from build123d import *

# Parameters (mm, degrees)
F1_DEPTH = 38.1
F2_R     = 19.05
F3_DEPTH = 101.601


with BuildPart() as f1:
    # F0 (on Top) → F1 (new body, symmetric)
    with BuildSketch(Plane.XY):
        Polygon((-50.8, -25.4), (50.8, -25.4), (50.8, 25.4), (25.4, 25.4), (0, 25.4), (-25.4, 25.4), (-50.8, 25.4), align=None)
        Polygon((0, 25.4), (25.4, 25.4), (25.4, 76.2), (-25.4, 76.2), (-25.4, 25.4), align=None)
    extrude(amount=F1_DEPTH, both=True)

    # F2 (on face) → F3 (cut, through all)
    with BuildSketch(Plane.YZ.offset(50.8)):
        Circle(F2_R)
    extrude(amount=-F3_DEPTH, mode=Mode.SUBTRACT)


solid = f1.part
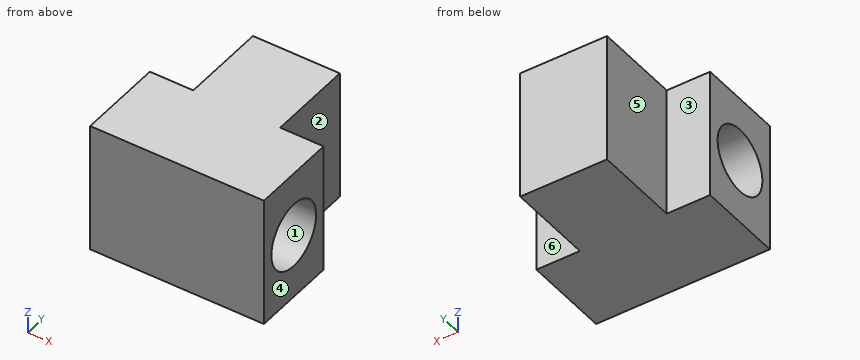
The model under review builds one solid part; all positions refer to its coordinate system, in mm. Face numbers are marked on the shaded views. A direction names the side the tool comes from. Round coordinates to 2 decimals unless told otherwise and drop trailing zeros. Order: outer loops, then holes, each group sorted by start corner. A loop starts at its lowest first (then second) coordinate and runs counter-clockwise, first axis right, second up. Notation, with made-up numbers: (83, -12) - (112, -12) arc R23 cw to (112, 4) - close; hole circle Ø7 at (27.25, 68). An arc over 180 degrees is marked (long way). Use one line per item in the form item = value.
Q1. Add section B-B on y = 0. Give the boundary of the cut face in (x, z), then the cut area to 3 significant figures.
Response values:
outline = (-50.8, -38.1) - (50.8, -38.1) - (50.8, -19.05) - (-50.8, -19.05) - close; (-50.8, 19.05) - (50.8, 19.05) - (50.8, 38.1) - (-50.8, 38.1) - close
area = 3,870 mm^2
Q2. To check wall thickness, follow line 1 (Z direction, x = -23, y = 0); line 2 (X direction, y = 43.5, z = 29); line 3 (Z direction, x = 14.5, y = -9). State the ranges of each line that lie inside material, in increasing order.
Response values:
line_1 = -38.1 to -19.05, 19.05 to 38.1
line_2 = -25.4 to 25.4
line_3 = -38.1 to -16.79, 16.79 to 38.1
Q3. Add section C-C on x = 5.5. Give the boundary of the cut face in (y, z), then the cut area to 3 significant figures.
Response values:
outline = (-25.4, -38.1) - (76.2, -38.1) - (76.2, 38.1) - (-25.4, 38.1) - close; hole circle Ø38.1 at (0, 0)
area = 6,600 mm^2
Q4. Tool access review of the marked faces 4, 5 and 6: name each direction out of +Z, -Z, +X, -X, +Y, -Y from which nothing blocks a thin tool from reaching the whole face with its end or side.
Response values:
face_4 = +Z, -Z, +X, +Y, -Y
face_5 = +Z, -Z, -X, +Y
face_6 = +Z, -Z, +X, +Y
Q5. Clearance check with flat-ended pins moving along their axes: P1, Ø15, axis at y = 49.5, z = -13.5, coming from the +X side; P2, Ø1.5, axis at y = -1, z = 17, coming from the +X side; P3, Ø12.5, axis at x = 37.5, z = -10.5, coming from the +Y side. State where each tip first meets the part, or that it passes through.
Response values:
P1 = 25.4
P2 = through
P3 = 25.4
Q6. Add section D-D on z = -20.5. Give the boundary of the cut face in (x, y).
Response values:
outline = (-50.8, -25.4) - (50.8, -25.4) - (50.8, 25.4) - (25.4, 25.4) - (25.4, 76.2) - (-25.4, 76.2) - (-25.4, 25.4) - (-50.8, 25.4) - close
Q7. Mouldability with a two-part tool opening along Y and no side actions: class the marked faces 1, 2 and 3 as pulls with the +Y half, pulls with the -Y half, needs draft (parallel to the pull), parting line crosses it, or undercut.
Response values:
face_1 = undercut
face_2 = needs draft
face_3 = pulls with the +Y half
Q8. Add section A-A on z = 0. Give the boundary of the cut face in (x, y).
Response values:
outline = (-50.8, -25.4) - (50.8, -25.4) - (50.8, -19.05) - (-50.8, -19.05) - close; (-50.8, 19.05) - (50.8, 19.05) - (50.8, 25.4) - (25.4, 25.4) - (25.4, 76.2) - (-25.4, 76.2) - (-25.4, 25.4) - (-50.8, 25.4) - close
